from build123d import *

# Parameters (mm, degrees)
F1_DEPTH = 0.8


# Not quite as in the source:
# - ends of sketch curves that miss each other by under 0.0002 mm in the source are joined


with BuildPart() as f1:
    # F0 (on Top) → F1 (new body, symmetric)
    with BuildSketch(Plane.XY):
        with BuildLine():
            Line((-13.5, 29.939975), (-13.5, 8.264975))
            ThreePointArc((-13.5, 8.264975), (0, -29.989975), (13.500000361, 8.2649754478))
            Line((13.500000361, 8.2649754478), (13.5, 29.939975))
            Line((13.5, 29.939975), (13.5, 29.964975))
            Line((13.5, 29.964975), (13.475, 29.964975))
            Line((13.475, 29.964975), (-13.475, 29.964975))
            Line((-13.475, 29.964975), (-13.5, 29.964975))
            Line((-13.5, 29.964975), (-13.5, 29.939975))
        make_face()
        with BuildLine():
            ThreePointArc((0, 9.564975), (18, -8.435025), (0, -26.435025))
            ThreePointArc((0, -26.435025), (-18, -8.435025), (0, 9.564975))
        make_face(mode=Mode.SUBTRACT)
    extrude(amount=F1_DEPTH, both=True)


solid = f1.part
The model under review builds one solid part; all positions refer to its coordinate system, in mm. Round coordinates to 2 decimals unless told otherwise and drop trailing zeros. Write each loop counter-clockwise with the first axis right and the second up, starting at its lowest first coordinate (ties: lowest second). Pieces come first, ordered by that corner, then holes. Notation, with made-up numbers: M 9.25,85 L 31.25,85 A19 ccw 31.25,115 Z; hole C 21,59 d8. An arc over 180 degrees is marked long. Use a Markdown table: item, result. Add a question column.
Q1. We need section D-D, the plane y = 14. State the section outline as (x, z) points, plus the area to 3 significant figures.
Q2. We need section C-C, the plane z = -0.1. State the section outline as (x, y) points.
Q3. The part is to be moulded in two halves that separate along X. For faces 1 (the face through (-0.742, -29.977, 0.011)), 2 (the face through (0, 14, 0.8)), 3 (the face through (-13.5, 19, 0)), 4 (the face through (10.95, 5.85, 0.01)), say which applies: pulls with the +X half, pulls with the -X half, needs draft (parallel to the pull), parting line crosses it, or undercut.
Q4. We need section A-A, the plane x = 0. State the section outline as (y, z) points, plus the area to 3 significant figures.
Q5. We need section B-B, the plane y = -2. State the section outline as (x, z) points, plus the area to 3 significant figures.
Q6. To check wall thickness, follow line 1 (Y direction, x = 0, z = -0.1); line 2 (X direction, y = -8.5, z = -0.55); line 3 (X direction, y = 16, z = 0.25). State the ranges of each line that lie inside material, in increasing order.
Q7. Insertion check: pin 1 (0.5 mm diameter, centred on y = 17.5, z = 0, fed in from +X); pin 2 (12 mm diameter, centred on x = -14, y = 8.5, fed in from +Z). Each pin has a flat end and moves straight along its axis. Give the tip position at first contact, or say it passes through.
Findings below:
| question | item | result |
|---|---|---|
| 1 | outline | M -13.5,-0.8 L 13.5,-0.8 L 13.5,0.8 L -13.5,0.8 Z |
| 1 | area | 43.2 mm² |
| 2 | outline | M -13.5,8.26 A21.51 ccw long 13.5,8.26 L 13.5,29.96 L -13.5,29.96 Z; hole C 0,-8.44 d36 |
| 3 | face 1 | parting line crosses it |
| 3 | face 2 | needs draft |
| 3 | face 3 | pulls with the -X half |
| 3 | face 4 | undercut |
| 4 | outline | M -29.99,-0.8 L -26.44,-0.8 L -26.44,0.8 L -29.99,0.8 Z; M 9.56,-0.8 L 29.96,-0.8 L 29.96,0.8 L 9.56,0.8 Z |
| 4 | area | 38.3 mm² |
| 5 | outline | M -20.51,-0.8 L -16.81,-0.8 L -16.81,0.8 L -20.51,0.8 Z; M 16.81,-0.8 L 20.51,-0.8 L 20.51,0.8 L 16.81,0.8 Z |
| 5 | area | 11.8 mm² |
| 6 | line 1 | y = -29.99 to -26.44, 9.56 to 29.96 |
| 6 | line 2 | x = -21.51 to -18, 18 to 21.51 |
| 6 | line 3 | x = -13.5 to 13.5 |
| 7 | pin 1 | stops at x = 13.5 |
| 7 | pin 2 | stops at z = 0.8 |
